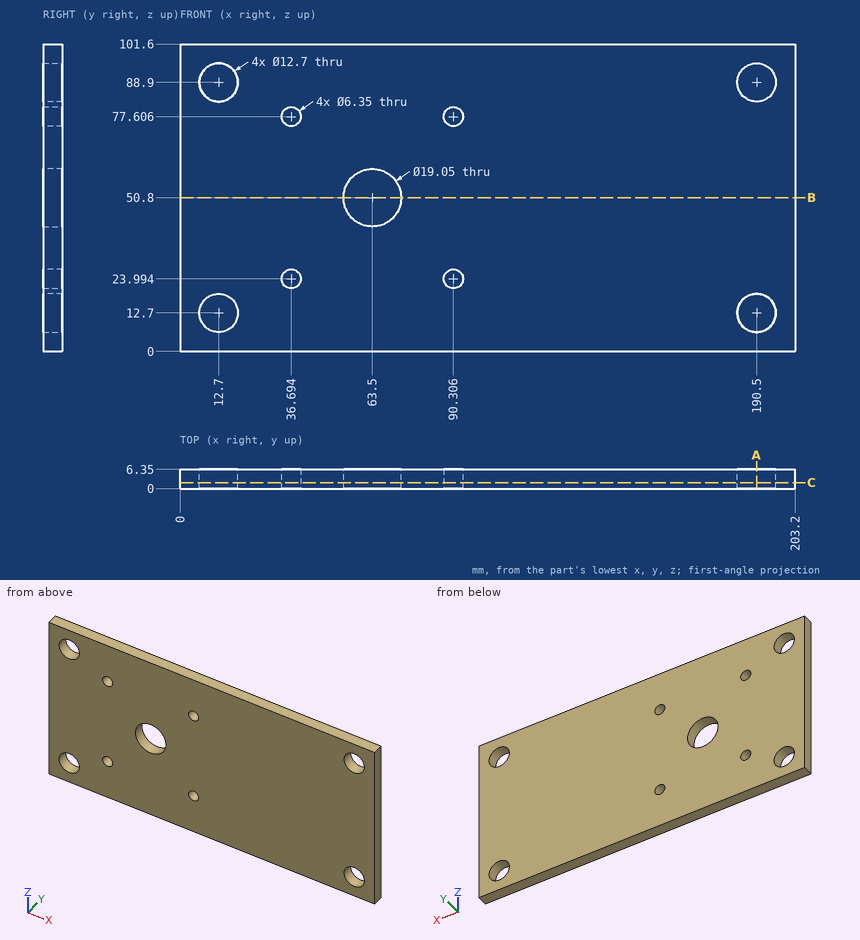
Drawing for the job (mm, zero at the part's lowest x, y, z). Coordinates: 2 decimals unless noted, no trailing zeros. Order: outer loops, then holes, each group sorted by start corner. A loop starts at its lowest first (then second) coordinate and runs counter-clockwise, first axis right, second up. Notation, with made-up numbers: (23, -13) -> (81, -13) arc R10 ccw to (81, 6) -> close; hole circle Ø10 at (7, 41.5). An arc over 180 degrees is marked (long way). One line per item, written item: value.
(1) Drop a flat-ended pin along its axis: pin 1 Ø10 at (x, z) = (190.5, 12.7) entering from -Y. Give the stop position or say it passes through.
Checked values:
pin 1: through
(2) Slice it at B-B, the plane z = 50.8. List the corners of the cut face in (x, y) (3 decimals), plus the area to 3 significant figures.
Checked values:
outline: (0, 0) -> (53.975, 0) -> (53.975, 6.35) -> (0, 6.35) -> close; (73.025, 0) -> (203.2, 0) -> (203.2, 6.35) -> (73.025, 6.35) -> close
area: 1,170 mm2
(3) Slice it at C-C, the plane y = 2. Count the separate pieces of the cut face and the enclosed holes in it, plus the area to 3 significant figures.
Checked values:
separate pieces: 1
enclosed holes: 9
area: 19,700 mm2
(4) Probe line 1 (X direction, y = 2.25, z = 88.9); line 2 (Z direction, x = 190.5, y = 5.25); line 3 (X direction, y = 4.25, z = 18.5) (1 decimal). List the from-to ranges inside material, lowest first. Write a range as [from, to].
Checked values:
line 1: [0, 6.35], [19.05, 184.15], [196.85, 203.2]
line 2: [0, 6.35], [19.05, 82.55], [95.25, 101.6]
line 3: [0, 10.1], [15.3, 187.9], [193.1, 203.2]
(5) Slice it at A-A, the plane x = 190.5. List the corners of the cut face in (y, z), plus the area to 3 significant figures.
Checked values:
outline: (0, 0) -> (6.35, 0) -> (6.35, 6.35) -> (0, 6.35) -> close; (0, 19.05) -> (6.35, 19.05) -> (6.35, 82.55) -> (0, 82.55) -> close; (0, 95.25) -> (6.35, 95.25) -> (6.35, 101.6) -> (0, 101.6) -> close
area: 484 mm2
